Source: CAD feature listing. Evaluate the final solid. Frame: model axes, mm. A direction names the side the tool comes from. Give positions to 0.01 mm unless a question says otherwise; leave off trailing zeros. Loops run counter-clockwise (first coordinate to the right, second up) from the corner with the lowest first, then second, coordinate; pieces in that order, holes last. Notation, with made-up numbers: M 33.5,-25 L 50.5,-25 A25 cw 50.5,-13 Z; hole C 0.25,2 d6. An arc over 180 degrees is marked long. Put each result on its own line as item: value.
Autodesk Inventor part; units mm, degrees
ref_plane "YZ Plane" through (0, 0, 0) normal (1, 0, 0) x (0, 1, 0)
ref_plane "XZ Plane" through (0, 0, 0) normal (0, 1, 0) x (-1, 0, 0)
ref_plane "XY Plane" through (0, 0, 0) normal (0, 0, 1) x (1, 0, 0)
sketch "Sketch1" plane through (0, 0, 0) normal (0, 0, 1) x (1, 0, 0)
  circle A0 centre (-16.8236, -8.8233) radius 2.1
  circle A1 centre (84.7764, -8.8233) radius 2.1
  circle A2 centre (84.7764, -59.6233) radius 2.1
  circle A3 centre (-16.8236, -59.6233) radius 2.1
  line L0 (-11.8121, -2.6233) -> (-16.8236, -2.6233)
  line L1 (84.7764, -65.7984) -> (79.7648, -65.7984)
  line L2 (90.9515, -41.9118) -> (90.9515, -51.9348)
  line L3 (-22.9988, -26.5348) -> (-22.9988, -16.5118)
  line L4 (-16.6488, -2.6233) -> (84.6015, -2.6233)
  line L5 (90.9515, -8.9733) -> (90.9515, -59.4484)
  line L6 (84.6015, -65.7984) -> (-16.6488, -65.7984)
  line L7 (-22.9988, -59.4484) -> (-22.9988, -8.9733)
  arc A4 (-16.6488, -2.6233) -> (-22.9988, -8.9733) centre (-16.6488, -8.9733) ccw
  arc A5 (-22.9988, -59.4484) -> (-16.6488, -65.7984) centre (-16.6488, -59.4484) ccw
  arc A6 (84.6015, -65.7984) -> (90.9515, -59.4484) centre (84.6015, -59.4484) ccw
  arc A7 (90.9515, -8.9733) -> (84.6015, -2.6233) centre (84.6015, -8.9733) ccw
  line L8 (-22.9988, -39.2857) -> (-21.9533, -40.3312)
  line L9 (-21.9533, -40.7802) -> (-22.9988, -41.8257)
  arc A8 (-21.9533, -40.7802) -> (-21.9533, -40.3312) centre (-22.1778, -40.5557) ccw
  line L10 (33.9764, -2.6233) -> (33.9764, -65.7984)
  line L11 (90.9515, -39.2857) -> (89.906, -40.3312)
  line L12 (89.906, -40.7802) -> (90.9515, -41.8257)
  arc A9 (89.906, -40.3312) -> (89.906, -40.7802) centre (90.1305, -40.5557) ccw
  point P0 (0, 0)
  point P1 (-22.9988, -2.6233)
  point P2 (90.9515, -65.7984)
  point P3 (90.9515, -2.6233)
  point P4 (-21.7288, -40.5557)
  dimension "d0" = 113.9502
  dimension "d1" = 63.1751
  dimension "d2" = 6.35
  dimension "d3" = 1.27
  dimension "d4" = 1.27
  dimension "d5" = 0.3175
extrude "Extrusion1" add sketch "Sketch1" along normal blind 4.318 contours L4 L10 L6 A5 L7 L9 A8 L8 L3 A4 L0 | L4 A7 L5 L11 A9 L12 L2 A6 L1 L6 L10
sketch "Sketch2" plane through (0, 0, 4.318) normal (0, 0, 1) x (1, 0, 0)
  point P0 (0, 0)
sketch "Sketch3" plane through (0, 0, 4.318) normal (0, 0, 1) x (1, 0, 0)
  line L0 (-11.0608, -23.7053) -> (-1.734, -23.7053) construction
  line L1 (-1.734, -23.7053) -> (-1.734, -28.4261) construction
  line L2 (-1.734, -28.4261) -> (-11.0608, -28.4261) construction
  line L3 (-11.0608, -28.4261) -> (-11.0608, -23.7053) construction
  line L4 (84.6015, -2.6233) -> (-16.6488, -2.6233) construction
  line L5 (33.9764, -2.6233) -> (33.9764, -66.312) construction
  line L6 (-22.9988, -8.9733) -> (-22.9988, -39.2857) construction
  line L7 (-22.9988, -34.4676) -> (90.982, -34.4676) construction
  line L8 (-3.8427, -43.7165) -> (8.5485, -43.7165)
  line L9 (8.5485, -43.7165) -> (7.9543, -46.5653)
  line L10 (7.9543, -46.5653) -> (-12.0569, -46.5653)
  line L11 (-12.0569, -46.5653) -> (-10.6937, -40.1512)
  spline S0 degree 2 poles (-10.6937, -40.1512) (-10.3267, -38.5258) (-7.9498, -36.5684) (-6.3594, -36.5684) knots 0 0 0 1 2 2 2
  line L12 (-6.3594, -36.5684) -> (2.449, -36.5684)
  line L13 (2.449, -36.5684) -> (4.5637, -26.589)
  line L14 (4.5637, -26.589) -> (-0.19, -26.589)
  line L15 (-0.19, -26.589) -> (-0.994, -30.3641)
  line L16 (-0.994, -30.3641) -> (-8.614, -30.3641)
  line L17 (-8.614, -30.3641) -> (-7.9848, -27.2881)
  spline S1 degree 2 poles (-7.9848, -27.2881) (-7.6178, -25.6627) (-5.2234, -23.7053) (-3.6505, -23.7053) knots 0 0 0 1 2 2 2
  line L18 (-3.6505, -23.7053) -> (9.2126, -23.7053)
  spline S2 degree 2 poles (9.2126, -23.7053) (10.838, -23.7053) (12.3935, -25.6627) (12.0264, -27.2881) knots 0 0 0 1 2 2 2
  line L19 (12.0264, -27.2881) -> (10.2263, -35.8344)
  spline S3 degree 2 poles (10.2263, -35.8344) (9.8768, -37.4597) (7.4824, -39.4172) (5.892, -39.4172) knots 0 0 0 1 2 2 2
  line L20 (5.892, -39.4172) -> (-2.9164, -39.4172)
  line L21 (-2.9164, -39.4172) -> (-3.8427, -43.7165)
  spline S4 degree 2 poles (14.8752, -27.2881) (15.2422, -25.6627) (17.6366, -23.7053) (19.2095, -23.7053) knots 0 0 0 1 2 2 2
  line L22 (19.2095, -23.7053) -> (32.0726, -23.7053)
  spline S5 degree 2 poles (32.0726, -23.7053) (33.698, -23.7053) (35.2535, -25.6627) (34.8864, -27.2881) knots 0 0 0 1 2 2 2
  line L23 (34.8864, -27.2881) -> (31.5658, -42.9825)
  spline S6 degree 2 poles (31.5658, -42.9825) (31.1988, -44.6079) (28.8219, -46.5653) (27.2315, -46.5653) knots 0 0 0 1 2 2 2
  line L24 (27.2315, -46.5653) -> (14.3859, -46.5653)
  spline S7 degree 2 poles (14.3859, -46.5653) (12.7605, -46.5653) (11.24, -44.6079) (11.572, -42.9825) knots 0 0 0 1 2 2 2
  line L25 (11.572, -42.9825) -> (11.7992, -41.7941)
  line L26 (11.7992, -41.7941) -> (19.4192, -41.7941)
  line L27 (19.4192, -41.7941) -> (19.0173, -43.7165)
  line L28 (19.0173, -43.7165) -> (23.7885, -43.7165)
  line L29 (23.7885, -43.7165) -> (24.7148, -39.4172)
  line L30 (24.7148, -39.4172) -> (15.9064, -39.4172)
  spline S8 degree 2 poles (15.9064, -39.4172) (14.281, -39.4172) (12.7255, -37.4597) (13.0925, -35.8344) knots 0 0 0 1 2 2 2
  line L31 (13.0925, -35.8344) -> (14.8752, -27.2881)
  line L32 (22.67, -26.589) -> (20.5378, -36.5684)
  line L33 (20.5378, -36.5684) -> (25.309, -36.5684)
  line L34 (25.309, -36.5684) -> (27.4237, -26.589)
  line L35 (27.4237, -26.589) -> (22.67, -26.589)
  spline S9 degree 2 poles (37.7352, -27.2881) (38.1022, -25.6627) (40.4966, -23.7053) (42.0695, -23.7053) knots 0 0 0 1 2 2 2
  line L36 (42.0695, -23.7053) -> (54.9326, -23.7053)
  spline S10 degree 2 poles (54.9326, -23.7053) (56.558, -23.7053) (58.1135, -25.6627) (57.7464, -27.2881) knots 0 0 0 1 2 2 2
  line L37 (57.7464, -27.2881) -> (54.4258, -42.9825)
  spline S11 degree 2 poles (54.4258, -42.9825) (54.0588, -44.6079) (51.6819, -46.5653) (50.0915, -46.5653) knots 0 0 0 1 2 2 2
  line L38 (50.0915, -46.5653) -> (37.2459, -46.5653)
  spline S12 degree 2 poles (37.2459, -46.5653) (35.6205, -46.5653) (34.1, -44.6079) (34.432, -42.9825) knots 0 0 0 1 2 2 2
  line L39 (34.432, -42.9825) -> (34.6592, -41.7941)
  line L40 (34.6592, -41.7941) -> (42.2792, -41.7941)
  line L41 (42.2792, -41.7941) -> (41.8773, -43.7165)
  line L42 (41.8773, -43.7165) -> (46.6485, -43.7165)
  line L43 (46.6485, -43.7165) -> (47.5748, -39.4172)
  line L44 (47.5748, -39.4172) -> (38.7664, -39.4172)
  spline S13 degree 2 poles (38.7664, -39.4172) (37.141, -39.4172) (35.5855, -37.4597) (35.9525, -35.8344) knots 0 0 0 1 2 2 2
  line L45 (35.9525, -35.8344) -> (37.7352, -27.2881)
  line L46 (45.53, -26.589) -> (43.3978, -36.5684)
  line L47 (43.3978, -36.5684) -> (48.169, -36.5684)
  line L48 (48.169, -36.5684) -> (50.2837, -26.589)
  line L49 (50.2837, -26.589) -> (45.53, -26.589)
  line L50 (71.3611, -39.4172) -> (69.8406, -46.5653)
  line L51 (69.8406, -46.5653) -> (62.2555, -46.5653)
  line L52 (62.2555, -46.5653) -> (63.776, -39.4172)
  line L53 (63.776, -39.4172) -> (60.8923, -23.7053)
  line L54 (60.8923, -23.7053) -> (68.5123, -23.7053)
  line L55 (68.5123, -23.7053) -> (70.662, -35.5023)
  line L56 (70.662, -35.5023) -> (77.7926, -23.7053)
  line L57 (77.7926, -23.7053) -> (80.8686, -23.7053)
  line L58 (80.8686, -23.7053) -> (71.3611, -39.4172)
  point P0 (0, 0)
  point P1 (-11.0608, -26.0657)
  dimension "d8" = 11.938
  dimension "d11" = 21.082
extrude "Extrusion3" add sketch "Sketch3" along normal blind 2.032
sketch "Sketch4" plane through (0, 0, 4.318) normal (0, 0, 1) x (1, 0, 0)
  line L0 (-22.9988, -39.2857) -> (-21.9533, -40.3312)
  line L1 (-21.9533, -40.7802) -> (-22.9988, -41.8257)
  arc A0 (-21.9533, -40.7802) -> (-21.9533, -40.3312) centre (-22.1778, -40.5557) ccw
  line L2 (90.9515, -41.8257) -> (89.906, -40.7802)
  arc A1 (89.906, -40.3312) -> (89.906, -40.7802) centre (90.1305, -40.5557) ccw
  line L3 (89.906, -40.3312) -> (90.9515, -39.2857)
  line L4 (-22.9988, -8.9733) -> (-22.9988, -39.2857) construction
  line L5 (-22.9988, -34.2082) -> (90.9515, -34.2082) construction
  line L6 (90.9515, -39.2857) -> (90.9515, -8.9733) construction
  line L7 (84.6015, -2.6233) -> (-16.6488, -2.6233) construction
  line L8 (-22.9988, -29.1307) -> (-21.9533, -28.0852)
  line L9 (-21.9533, -27.6362) -> (-22.9988, -26.5907)
  arc A2 (-21.9533, -28.0852) -> (-21.9533, -27.6362) centre (-22.1778, -27.8607) ccw
  line L10 (90.9515, -26.5907) -> (89.906, -27.6362)
  arc A3 (89.906, -27.6362) -> (89.906, -28.0852) centre (90.1305, -27.8607) ccw
  line L11 (89.906, -28.0852) -> (90.9515, -29.1307)
  line L12 (90.9515, -26.5907) -> (90.9515, -29.1307) construction
  line L13 (-22.9988, -26.5907) -> (-22.9988, -29.1307) construction
  line L14 (-22.9988, -26.5907) -> (-22.9988, -29.1307)
  line L15 (90.9515, -26.5907) -> (90.9515, -29.1307)
  point P0 (0, 0)
  dimension "d14" = 31.5849
extrude "Extrusion4" cut sketch "Sketch4" against normal through all
sketch "Sketch5" plane through (0, 0, 4.318) normal (0, 0, 1) x (1, 0, 0)
  circle A0 centre (-16.8236, -8.8233) radius 2.1
  circle A1 centre (-16.8236, -8.8233) radius 2.3368
  circle A2 centre (84.7764, -8.8233) radius 2.1
  circle A3 centre (84.7764, -59.6233) radius 2.1
  circle A4 centre (-16.8236, -59.6233) radius 2.1
  circle A5 centre (84.7764, -8.8233) radius 2.3368
  circle A6 centre (84.7764, -59.6233) radius 2.3368
  circle A7 centre (-16.8236, -59.6233) radius 2.3368
  point P0 (0, 0)
  dimension "d17" = 4.6736
  dimension "d18" = 4.6736
  dimension "d19" = 4.6736
  dimension "d20" = 4.6736
extrude "Extrusion5" cut sketch "Sketch5" against normal blind 25.4
properties part number "299Y"
1. Material intervals for line 1 (X direction, y = -61.5, z = 3.5); line 2 (X direction, y = -40, z = 5.5); line 3 (Y direction, x = 20, z = 6), sorted ascending. Write a range as from..to.
Found:
line 1: -22.66..-18.22, -15.43..83.38, 86.17..90.61
line 2: -10.66..-3.04, 24.59..32.2, 47.45..55.06, 63.65..71.24
line 3: -46.57..-43.72, -39.42..-23.71
2. Draft query along X for faces 1 (the flat face through (2, -26.589, 5)), 2 (the flat face through (-22.999, -34, 2)), 3 (the flat face through (48, -23.705, 5)). Return one class per face: pulls with the +X half, pulls with the -X half, needs draft (parallel to the pull), parting line crosses it, or undercut.
Found:
face 1: undercut
face 2: pulls with the -X half
face 3: needs draft
3. Access query for faces 4 (the flat face through (43, -39.417, 5)), 5 (the flat face through (-2, -36.568, 5)), 6 (the flat face through (13.97, -31.62, 5.32)), 7 (the flat face through (66, -46.565, 5)). Directions: +Z, -Z, +X, -X, +Y, -Y. A direction counts if a zero-diameter tool reaches every point of the face in a straight line with its end or side. Return the directions, or none.
Found:
face 4: +Z
face 5: +Z, -X
face 6: +Z, +Y
face 7: +Z, +X, -X, -Y
4. Contact query for flat-ended pins moving along their axis: P1, Ø0.6, axis at x = 42, z = 5, coming from the -Y side; P2, Ø7.5, axis at x = -16.82, y = -59.62, coming from the +Z side; P3, Ø2, axis at x = 64, z = 6, coming from the +Y side. Output: stop coordinate, or through.
Found:
P1: y = -46.57
P2: z = 4.32
P3: y = -23.71
5. Section query B-B (y = -55). Output: boundary loops of the cut face in (x, z).
Found:
outline: M -23,0 L 90.95,0 L 90.95,4.32 L -23,4.32 Z
6. Section query A-A (z = 2.5). Output: boundary loops of the cut face in (x, y).
Found:
outline: M -23,-59.45 A6.35 ccw -16.65,-65.8 L 84.6,-65.8 A6.35 ccw 90.95,-59.45 L 90.95,-41.83 L 89.91,-40.78 A0.32 cw 89.91,-40.33 L 90.95,-39.29 L 90.95,-29.13 L 89.91,-28.09 A0.32 cw 89.91,-27.64 L 90.95,-26.59 L 90.95,-8.97 A6.35 ccw 84.6,-2.62 L -16.65,-2.62 A6.35 ccw -23,-8.97 L -23,-26.59 L -21.95,-27.64 A0.32 cw -21.95,-28.09 L -23,-29.13 L -23,-39.29 L -21.95,-40.33 A0.32 cw -21.95,-40.78 L -23,-41.83 Z; hole C -16.82,-59.62 d4.67; hole C -16.82,-8.82 d4.67; hole C 84.78,-59.62 d4.67; hole C 84.78,-8.82 d4.67
